Autodesk Inventor part; units mm, degrees
ref_plane "YZ Plane" through (0, 0, 0) normal (1, 0, 0) x (0, 1, 0)
ref_plane "XZ Plane" through (0, 0, 0) normal (0, 1, 0) x (-1, 0, 0)
ref_plane "XY Plane" through (0, 0, 0) normal (0, 0, 1) x (1, 0, 0)
sketch "Sketch1" plane through (0, 0, 0) normal (0, 0, 1) x (1, 0, 0)
  circle A0 centre (0, 0) radius 12.7
  line L0 (-6.35, -6.35) -> (6.35, -6.35)
  line L1 (6.35, -6.35) -> (6.35, 6.35)
  line L2 (6.35, 6.35) -> (-6.35, 6.35)
  line L3 (-6.35, 6.35) -> (-6.35, -6.35)
  point P0 (-6.35, 0)
  point P1 (0, 6.35)
  dimension "d0" = 25.4
  dimension "d1" = 12.7
  dimension "d2" = 12.7
extrude "Extrusion1" add sketch "Sketch1" against normal blind 152.4 contours A0 | L3 L2 L1 L0
extrude "Extrusion2" add sketch "Sketch1" along normal blind 12.7 contours L3 L2 L1 L0
sketch "Sketch2" plane through (6.35, -6.35, 12.7) normal (1, 0, 0) x (0, 0, -1)
  point P0 (12.7, 6.35)
  point P1 (6.35, 6.35)
hole "Hole1" at (6.35, 0, 6.35) direction (-1, 0, 0) diameter 9.525 depth 25.4 tip angle 118
thread "Thread1"
sketch "Sketch3" plane through (0, 0, -152.4) normal (0, 0, -1) x (-1, 0, 0)
  circle A0 centre (0, 0) radius 12.7
  circle A1 centre (0, 0) radius 3.175
  dimension "d16" = 6.35
extrude "Extrusion3" add sketch "Sketch3" along normal blind 101.6 contours A1
sketch "Sketch4" plane through (0, 0, -254) normal (0, 0, -1) x (-1, 0, 0)
  circle A0 centre (0, 0) radius 3.175
  line L0 (-3.175, -3.175) -> (3.175, -3.175)
  line L1 (3.175, -3.175) -> (3.175, 3.175)
  line L2 (3.175, 3.175) -> (-3.175, 3.175)
  line L3 (-3.175, 3.175) -> (-3.175, -3.175)
extrude "Extrusion4" add sketch "Sketch4" along normal blind 12.7
sketch "Sketch5" plane through (3.175, 0, -254) normal (1, 0, 0) x (0, 0, -1)
  line L0 (0, -3.175) -> (12.7, -3.175)
  point P0 (0, 0)
  point P1 (-254, 0)
  point P2 (6.35, 0)
  point P3 (6.35, -3.175)
hole "Hole2" at (3.175, 0, -260.35) direction (-1, 0, 0) diameter 3.175 depth 25.4 tip angle 118
properties part number "temp_cylinder_.1inch_4stroke"
Input: part model. Units: mm. Frame: model coordinates. A direction names the side the tool comes from. Coordinates: 2 decimals unless noted, no trailing zeros. Loops run counter-clockwise (first coordinate to the right, second up) from the corner with the lowest first, then second, coordinate; pieces in that order, holes last. Notation, with made-up numbers: (62, -2) - (89, -2) arc R12 cw to (89, 11) - close; hole circle Ø5 at (18.5, 88.5). An arc over 180 degrees is marked (long way). Answer in a Markdown table with one row per item. Add a question column.
Item 1: Mould query, pull axis Z, two halves, no side actions, for faces 1 (the cylindrical face through (0.69, 3.1, -202.49)), 2 (the cylindrical face through (-2.75, -12.4, -75.13)), 3 (the flat face through (0, 0, 12.7)). Classes: released by +Z, released by -Z, zero draft, split by the parting line, or undercut.
Item 2: Section query D-D on z = -155.5. Return the cut outline in (x, y) (3 decimals).
Item 3: Section query C-C on y = 10. Return the cut outline in (x, z).
Item 4: Contact query for flat-ended pins moving along their axis: P1, Ø5, axis at x = 1, z = -260, coming from the +Y side (3 decimals); P2, Ø11, axis at y = 0, z = 6.35, coming from the -X side; P3, Ø6, axis at y = 9, z = -102.5, coming from the -X side. Output: stop coordinate, or through.
Item 5: Line query: line 1 along Z through (x, y) = (0, 0); line 2 along Y through (x, z) = (0, 6.35); line 3 along Y through (x, z) = (0.25, -260.35) (1 decimal). Output: solid intervals per line, ascending. Write a range as [from, to].
Item 6: Section query B-B on z = -24. Return the cut outline in (x, y).
Item 7: Access query for faces 4 (the flat face through (6.35, 3, 2)), 5 (the flat face through (-3.175, -0.8, -258.8)), 6 (the flat face through (3.175, 0.8, -258.8)), 7 (the flat face through (0, -6.35, 6)). Directions: +Z, -Z, +X, -X, +Y, -Y. A direction counts if a zero-diameter tool reaches every point of the face in a straight line with its end or side. Return the directions, or none.
Item 8: Section query A-A on z = 6.35. Return the cut outline in (x, y), then the cut area to 3 significant figures.
Recorded:
| question | item | result |
|---|---|---|
| 1 | face 1 | undercut |
| 1 | face 2 | zero draft |
| 1 | face 3 | released by +Z |
| 2 | outline | circle Ø6.35 at (0, 0) |
| 3 | outline | (-7.83, -152.4) - (7.83, -152.4) - (7.83, 0) - (-7.83, 0) - close |
| 4 | P1 | y = 3.175 |
| 4 | P2 | x = -6.35 |
| 4 | P3 | x = -11.19 |
| 5 | line 1 | [-266.7, -261.94], [-258.76, 1.59], [11.11, 12.7] |
| 5 | line 2 | [-6.35, -4.76], [4.76, 6.35] |
| 5 | line 3 | [-3.2, -1.6], [1.6, 3.2] |
| 6 | outline | circle Ø25.4 at (0, 0) |
| 7 | face 4 | +Z, +X, +Y, -Y |
| 7 | face 5 | -Z, -X, +Y, -Y |
| 7 | face 6 | -Z, +X, +Y, -Y |
| 7 | face 7 | +Z, +X, -X, -Y |
| 8 | outline | (-6.35, -6.35) - (6.35, -6.35) - (6.35, -4.76) - (-6.35, -4.76) - close; (-6.35, 4.76) - (6.35, 4.76) - (6.35, 6.35) - (-6.35, 6.35) - close |
| 8 | area | 40.3 mm^2 |
